Read the model definition and answer for the solid it produces. Units are mm, in the model's axes. Coordinates: 2 decimals unless noted, no trailing zeros. Write each loop counter-clockwise with the first axis right and the second up, starting at its lowest first coordinate (ties: lowest second). Pieces come first, ordered by that corner, then holes. Notation, with made-up numbers: (15, -20) -> (58, -20) arc R13 cw to (58, -2) -> close; hole circle Ø8 at (38.5, -33.5). An arc over 180 degrees is marked (long way). Answer as a JSON object with one key per item and string values. Group by question number.
(1) Straight lines are drawn through the part: L1, parallel to Z at x = -728.5, y = 11; L2, parallel to X at y = -0.5, z = -6.25; L3, parallel to Z at x = 809, y = 1.5. For each, find the intervals that lie inside material, in ascending order.
(2) Flat-ended cylindrical pins translate along their axes: P1, Ø1, axis at x = 521, y = 5, coming from the +Z side; P2, Ø6, axis at y = 5.5, z = 8.5, coming from the -X side (3 decimals); P3, Ø5, axis at y = 6.5, z = 9.5, coming from the -X side (3 decimals); P4, Ø10, axis at x = -591.5, z = 10, coming from the +Y side (3 decimals). Find the tip coordinate at first contact, or state that the pin passes through.
(3) Find section A-A (x = -54.5). Give the vertices of the cut face in (y, z) (1 decimal), then the cut area to 3 significant figures.
from build123d import *

# Parameters (mm, degrees)
F1_DEPTH = 889
F2_SIZE  = 31.74999


# Not quite as in the source:
# - a fillet or chamfer is up to 0.001 mm smaller than in the source, because OpenCascade refuses the exact size


with BuildPart() as f1:
    # F0 (on Right) → F1 (new body, symmetric)
    with BuildSketch(Plane.YZ):
        with BuildLine():
            Line((-15.875, -14.2875), (15.875, -14.2875))
            Line((15.875, -14.2875), (15.875, 9.525))
            ThreePointArc((15.875, 9.525), (12.4385421004, 14.0991686237), (7.08843051, 12.07220847))
            ThreePointArc((7.08843051, 12.07220847), (5.9853917743, 11.4055483551), (4.789455264, 11.886033552))
            ThreePointArc((4.789455264, 11.886033552), (2.3755826554, 13.6595328458), (-0.5531949, 14.2875))
            Line((-0.5531949, 14.2875), (-15.875, 14.2875))
            Line((-15.875, 14.2875), (-15.875, -14.2875))
        make_face()
    extrude(amount=F1_DEPTH, both=True)

    # F2 (size 31.75 in the source; OpenCascade refuses exactly that, so slightly less here)
    f2_edges = [f1.edges().sort_by_distance(p)[0] for p in [
        (-889, -15.875, 0),
        (889, -15.875, 0),
    ]]
    chamfer(f2_edges, length=F2_SIZE)


solid = f1.part
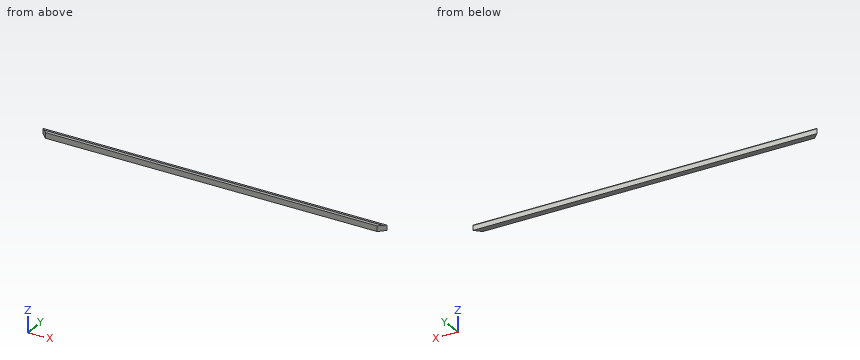
Results below:
{
 "1": {"L1": "z = -14.29 to 14.29", "L2": "x = -872.63 to 872.63", "L3": "z = -14.29 to 13.99"},
 "2": {"P1": "stops at z = 12.19", "P2": "stops at x = -881.625", "P3": "stops at x = -882.125", "P4": "stops at y = 15.875"},
 "3": {"outline": "(-15.9, -14.3) -> (15.9, -14.3) -> (15.9, 9.5) arc R4.8 ccw to (7.1, 12.1) arc R1.4 cw to (4.8, 11.9) arc R7.1 ccw to (-0.6, 14.3) -> (-15.9, 14.3) -> close", "area": "890 mm2"}
}
